Part model, mm, in its own coordinate system. Coordinates: 2 decimals unless noted, no trailing zeros. Order: outer loops, then holes, each group sorted by start corner. A loop starts at its lowest first (then second) coordinate and runs counter-clockwise, first axis right, second up. Notation, with made-up numbers: (34.5, 13.5) - (57.5, 13.5) arc R27 cw to (57.5, 44.5) - close; hole circle Ø5 at (-16, 64). An arc over 180 degrees is marked (long way). Use a Markdown table: item, result. Add a question column.
1) Drop a flat-ended pin along its axis: P1, Ø1, axis at y = 307.5, z = 3, coming from the -X side. Give the stop position or say it passes through.
2) Wall check: L1, parallel to Y at x = 95, z = 3.7; L2, parallel to X at y = 283, z = 2.75; L3, parallel to X at y = 315.5, z = 1.65. Give the ranges that are in metal, low to high. Write a range as [from, to].
3) Saw through at B-B on z = 1.8. List the corners of the cut face in (x, y) (1 decimal), then the cut area to 3 significant figures.
4) Saw through at A-A on y = 101.6. List the corners of the cut face in (x, z).
5) Two-plate mould, pull along Y, no slides. Class faces 1 (the face through (27.616, 5.653, 2.317)), 2 (the face through (70.6, 202.68, 2.32)), 3 (the face through (50, 193, 0)): +Y half, -Y half, draft (parallel to the pull), parting line (faces both ways), or undercut.
6) Saw through at C-C on x = 9.5. List the corners of the cut face in (y, z), then the cut area to 3 significant figures.
7) Saw through at D-D on y = 183. List the corners of the cut face in (x, z), then the cut area to 3 significant figures.
```python
from build123d import *

# Parameters (mm, degrees)
F0_R        = 5.08
F1_DEPTH    = 4.699
F2_T1_DEPTH = 25.7410489686
F2_T3_DEPTH = 55.499


# Not quite as in the source:
# - a fillet or chamfer that OpenCascade refuses, or shapes differently, is made with other operations: its cross-section is extruded or revolved along the edge and cut away or added


with BuildPart() as f1:
    # F0 (on Top) → F1 (new body)
    with BuildSketch(Plane.XY):
        with BuildLine():
            Line((31.4325, 165.1), (1.5875, 165.1))
            ThreePointArc((1.5875, 165.1), (1.1225320151, 163.9774679849), (0, 163.5125))
            Line((0, 163.5125), (0, 19.05))
            Line((0, 19.05), (19.05, 0))
            Line((19.05, 0), (33.02, 0))
            Line((33.02, 0), (33.02, 163.5125))
            ThreePointArc((33.02, 163.5125), (31.8974679849, 163.9774679849), (31.4325, 165.1))
        make_face()
        with Locations((25.2715107054, 10.16)):
            Circle(F0_R, mode=Mode.SUBTRACT)
        with Locations((24.5934482664, 101.6)):
            Circle(F0_R, mode=Mode.SUBTRACT)
        with BuildLine():
            Line((76.2, 368.6610758305), (76.2, 242.8875))
            ThreePointArc((76.2, 242.8875), (77.3225320151, 242.4225320151), (77.7875, 241.3))
            Line((77.7875, 241.3), (92.71, 241.3))
            Line((92.71, 241.3), (92.71, 277.1550263596))
            ThreePointArc((92.71, 277.1550263596), (87.63, 282.2350263596), (92.71, 287.3150263596))
            Line((92.71, 287.3150263596), (92.71, 356.975927515))
            ThreePointArc((92.71, 356.975927515), (87.63, 362.055927515), (92.71, 367.135927515))
            Line((92.71, 367.135927515), (92.71, 384.755953431))
            ThreePointArc((92.71, 384.755953431), (81.1825763095, 380.0653413474), (76.2, 368.6610758305))
        make_face()
        with BuildLine():
            Line((92.71, 277.1550263596), (92.71, 241.3))
            Line((92.71, 241.3), (107.6325, 241.3))
            ThreePointArc((107.6325, 241.3), (108.0974679849, 242.4225320151), (109.22, 242.8875))
            Line((109.22, 242.8875), (109.22, 368.8926994801))
            ThreePointArc((109.22, 368.8926994801), (104.1590146553, 380.148561327), (92.71, 384.755953431))
            Line((92.71, 384.755953431), (92.71, 367.135927515))
            ThreePointArc((92.71, 367.135927515), (96.3021024484, 365.6480299635), (97.79, 362.055927515))
            ThreePointArc((97.79, 362.055927515), (96.3021024484, 358.4638250666), (92.71, 356.975927515))
            Line((92.71, 356.975927515), (92.71, 287.3150263596))
            ThreePointArc((92.71, 287.3150263596), (96.3021024484, 285.827128808), (97.79, 282.2350263596))
            ThreePointArc((97.79, 282.2350263596), (96.3021024484, 278.6429239111), (92.71, 277.1550263596))
        make_face()
        with BuildLine():
            ThreePointArc((1.1225320151, 166.2225320151), (1.4666587579, 165.7075099489), (1.5875, 165.1))
            Line((1.5875, 165.1), (31.4325, 165.1))
            ThreePointArc((31.4325, 165.1), (32.4124900511, 166.5666587579), (34.1425320151, 166.2225320151))
            Line((34.1425320151, 166.2225320151), (108.0974679849, 240.1774679849))
            ThreePointArc((108.0974679849, 240.1774679849), (107.7533412421, 240.6924900511), (107.6325, 241.3))
            Line((107.6325, 241.3), (92.71, 241.3))
            Line((92.71, 241.3), (77.7875, 241.3))
            ThreePointArc((77.7875, 241.3), (76.8075099489, 239.8333412421), (75.0774679849, 240.1774679849))
            Line((75.0774679849, 240.1774679849), (1.1225320151, 166.2225320151))
        make_face()
    extrude(amount=F1_DEPTH)

    # F2: fillet of radius 10.16 on 3 edges, made by hand

    # F2_s2 → F2_t1 (cut)
    with BuildSketch(Plane.XY.offset(-10.5210244843)):
        with BuildLine():
            ThreePointArc((0, 23.2584097937), (0.7733839497, 19.3703461209), (2.9757951031, 16.0742048969))
            Line((2.9757951031, 16.0742048969), (0, 19.05))
            Line((0, 19.05), (0, 23.2584097937))
        make_face()
        with BuildLine():
            ThreePointArc((16.0742048969, 2.9757951031), (19.3703461209, 0.7733839497), (23.2584097937, 0))
            Line((23.2584097937, 0), (19.05, 0))
            Line((19.05, 0), (16.0742048969, 2.9757951031))
        make_face()
    extrude(amount=F2_T1_DEPTH, mode=Mode.SUBTRACT)

    # F2_s4 → F2_t3 (cut)
    with BuildSketch(Plane.XY.offset(-25.4)):
        with BuildLine():
            ThreePointArc((22.86, 0), (30.0442048969, 2.9757951031), (33.02, 10.16))
            Line((33.02, 10.16), (33.02, 0))
            Line((33.02, 0), (22.86, 0))
        make_face()
    extrude(amount=F2_T3_DEPTH, mode=Mode.SUBTRACT)


solid = f1.part
```
Results are:
| question | item | result |
|---|---|---|
| 1 | P1 | x = 76.2 |
| 2 | L1 | [227.08, 277.7], [286.77, 357.52], [366.59, 384.6] |
| 2 | L2 | [76.2, 87.69], [97.73, 109.22] |
| 2 | L3 | [76.2, 109.22] |
| 3 | outline | (0, 23.3) arc R10.2 ccw to (3, 16.1) - (16.1, 3) arc R10.2 ccw to (23.1, 0) arc R10.2 ccw to (33, 10.2) - (33, 163.5) arc R1.6 cw (long way) to (34.1, 166.2) - (108.1, 240.2) arc R1.6 cw to (109.2, 242.9) - (109.2, 368.9) arc R16.5 ccw to (76.2, 368.7) - (76.2, 242.9) arc R1.6 cw (long way) to (75.1, 240.2) - (1.1, 166.2) arc R1.6 cw to (0, 163.5) - close; hole circle Ø10.2 at (24.6, 101.6); hole circle Ø10.2 at (25.3, 10.2); hole circle Ø10.2 at (92.7, 282.2); hole circle Ø10.2 at (92.7, 362.1) |
| 3 | area | 12,000 mm2 |
| 4 | outline | (0, 0) - (19.51, 0) - (19.51, 4.7) - (0, 4.7) - close; (29.67, 0) - (33.02, 0) - (33.02, 4.7) - (29.67, 4.7) - close |
| 5 | face 1 | undercut |
| 5 | face 2 | -Y half |
| 5 | face 3 | draft |
| 6 | outline | (9.55, 0) - (174.6, 0) - (174.6, 4.7) - (9.55, 4.7) - close |
| 6 | area | 776 mm2 |
| 7 | outline | (17.9, 0) - (50.92, 0) - (50.92, 4.7) - (17.9, 4.7) - close |
| 7 | area | 155 mm2 |
